Read the model definition and answer for the solid it produces. Units are mm, in the model's axes. A direction names the side the tool comes from. Coordinates: 2 decimals unless noted, no trailing zeros. Order: outer loops, then holes, each group sorted by start corner. A loop starts at its lowest first (then second) coordinate and runs counter-clockwise, first axis right, second up. Notation, with made-up numbers: (5.5, 59.25) - (27.5, 59.25) arc R16 cw to (27.5, 74.25) - close; hole circle Ø9 at (-27.5, -12.5). An arc over 180 degrees is marked (long way). Use one line per item in the form item = value.
Autodesk Inventor part; units mm, degrees
ref_plane "YZ Plane" through (0, 0, 0) normal (1, 0, 0) x (0, 1, 0)
ref_plane "XZ Plane" through (0, 0, 0) normal (0, 1, 0) x (-1, 0, 0)
ref_plane "XY Plane" through (0, 0, 0) normal (0, 0, 1) x (1, 0, 0)
sketch "Sketch1" plane through (0, 0, 0) normal (1, 0, 0) x (0, 1, 0)
  line L0 (0, 0) -> (12.7, 0)
  circle A0 centre (12.7, 0) radius 2.1209
  circle A1 centre (0, 0) radius 2.1209
  line L1 (12.7, 0) -> (12.7, 6.35)
  line L2 (12.7, 6.35) -> (19.05, 6.35)
  line L3 (19.05, 6.35) -> (-6.35, 6.35)
  line L4 (-6.35, 6.35) -> (-6.35, -6.35)
  line L5 (-6.35, -6.35) -> (19.05, -6.35)
  line L6 (19.05, -6.35) -> (19.05, 6.35)
  line L7 (19.05, -6.35) -> (19.05, -19.05)
  line L8 (19.05, -19.05) -> (31.75, -19.05)
  line L9 (31.75, -19.05) -> (31.75, -6.35)
  line L10 (31.75, -6.35) -> (19.05, 6.35)
  line L11 (19.05, -19.05) -> (6.35, -6.35)
  line L12 (19.05, -12.7) -> (25.4, -12.7)
  circle A2 centre (25.4, -12.7) radius 2.1082
  line L13 (0, 0) -> (0, -44.45)
  circle A3 centre (0, -44.45) radius 2.1209
  line L14 (-6.35, -6.35) -> (31.75, -6.35)
  line L15 (31.75, -6.35) -> (31.75, -50.8)
  line L16 (31.75, -50.8) -> (-6.35, -50.8)
  line L17 (-6.35, -50.8) -> (-6.35, -6.35)
  line L18 (6.35, -6.35) -> (6.35, -50.8)
  line L19 (19.05, -19.05) -> (6.35, -19.05)
  line L20 (31.75, -6.35) -> (31.75, 15.3303)
  line L21 (31.75, 15.3303) -> (28.0303, 15.3303)
  line L22 (31.75, 15.3303) -> (34.925, 15.3303)
  line L23 (31.75, -19.05) -> (34.925, -19.05)
  line L24 (34.925, -19.05) -> (34.925, 15.3303)
  line L25 (28.0303, 15.3303) -> (19.05, 15.3303)
  line L26 (19.05, 15.3303) -> (19.05, 6.35)
  line L27 (34.925, 10.8401) -> (19.05, 10.8401)
  circle A4 centre (26.9875, 10.8401) radius 2.1209
  dimension "d0" = 12.7
  dimension "d1" = 4.2418
  dimension "d2" = 4.2418
  dimension "d3" = 6.35
  dimension "d4" = 6.35
  dimension "d5" = 25.4
  dimension "d6" = 12.7
  dimension "d7" = 12.7
  dimension "d8" = 4.2164
  dimension "d11" = 44.45
  dimension "d15" = 12.7
  dimension "d19" = 3.175
  dimension "d20" = 4.2418
extrude "Extrusion1" add sketch "Sketch1" along normal blind 3.175 contours A1 L13 L5 L4 L3 L1 A0 L0 | L0 A0 L1 L2 L6 L5 L13 A1 | L5 L18 L16 L17 | L5 L7 L11 | L11 L19 L18 | L14 L9 L8 L7 | L6 L10 L14 | L26 L27 A4 L20 L10 | L26 L25 L21 L20 L27 A4
fillet "Fillet1" radius 50.8 1 edges at (1.5875, 6.35, -19.05)
fillet "Fillet3" radius 3.175 6 edges at (1.5875, 31.75, 15.3303) (1.5875, 31.75, -19.05) (1.5875, 6.35, -50.8) (1.5875, -6.35, -50.8) (1.5875, -6.35, 6.35) (1.5875, 19.05, 15.3303)
fillet "Fillet4" radius 12.7 1 edges at (1.5875, 19.05, 6.35)
properties part number "sled mounts"
(1) The mould has two halves that part along Y. Classify faces 1 (the cylindrical face through (1.57, 14.72, -0.64)), 2 (the cylindrical face through (1.6, 31.3, -18.8)), 3 (the flat face through (2, -6.35, -22)): +Y half, -Y half, draft (parallel to the pull), parting line (faces both ways), or undercut.
Answer list:
face_1 = undercut
face_2 = +Y half
face_3 = -Y half
(2) Section A-A, the plane z = -12.7 is taken. Write down the section's boundary in (x, y) (3 decimals).
Answer list:
outline = (0, -6.35) - (3.175, -6.35) - (3.175, 23.292) - (0, 23.292) - close; (0, 27.508) - (3.175, 27.508) - (3.175, 31.75) - (0, 31.75) - close
(3) Straight lines are drawn through the part: L1, parallel to Z at x = 1.55, y = 0; L2, parallel to Y at x = 2.25, z = 0; L3, parallel to Z at x = 0.8, y = 25.4. For each, find the intervals that lie inside material, in ascending order.
Answer list:
L1 = -50.8 to -46.57, -42.33 to -2.12, 2.12 to 6.35
L2 = -6.35 to -2.12, 2.12 to 10.58, 14.82 to 31.75
L3 = -23.01 to -14.81, -10.59 to 9.43, 12.25 to 15.33
(4) Given pin 1 Ø7 at (y, z) = (0, 0) entering from -X; pin 2 Ø4 at (y, z) = (0, -44.45) entering from +X; pin 3 Ø1.5 at (x, y) = (3, 24.5) entering from -Z; pin 4 Ø1 at (x, y) = (1, 2) entering from +Z, each flat-ended and moving along its own axis, determine where each tip first touches the part or whether it passes through.
Answer list:
pin_1 = 0
pin_2 = through
pin_3 = -24.27
pin_4 = 6.35
(5) Which of the six approach directions +Z, -Z, +X, -X, +Y, -Y give full straight-line access (tool end or side, diameter ignored) to faces 4 (the flat face through (2, 2, 6.35)), 5 (the cylindrical face through (1.61, 30.84, 14.38))?
Answer list:
face_4 = +Z, +X, -X, -Y
face_5 = +Z, +X, -X, +Y
(6) Section B-B, the plane y = 0 is taken. Write down the section's boundary in (x, z) (3 decimals), then the cut area to 3 significant figures.
Answer list:
outline = (0, -50.8) - (3.175, -50.8) - (3.175, -46.571) - (0, -46.571) - close; (0, -42.329) - (3.175, -42.329) - (3.175, -2.121) - (0, -2.121) - close; (0, 2.121) - (3.175, 2.121) - (3.175, 6.35) - (0, 6.35) - close
area = 155 mm2
(7) Section D-D, the plane x = 0.75 is taken. State how many separate pieces and enclosed holes the cut face has, then the cut area to 3 significant figures.
Answer list:
separate_pieces = 1
enclosed_holes = 5
area = 1,710 mm2
(8) Section C-C, the plane z = 0 is taken. Write down the section's boundary in (x, y) (3 decimals), then the cut area to 3 significant figures.
Answer list:
outline = (0, -6.35) - (3.175, -6.35) - (3.175, -2.121) - (0, -2.121) - close; (0, 2.121) - (3.175, 2.121) - (3.175, 10.579) - (0, 10.579) - close; (0, 14.821) - (3.175, 14.821) - (3.175, 31.75) - (0, 31.75) - close
area = 94.0 mm2
